Part model, mm, in its own coordinate system. Face numbers are marked on the shaded views. A direction names the side the tool comes from. Round coordinates to 2 decimals unless told otherwise and drop trailing zeros. Loops run counter-clockwise (first coordinate to the right, second up) from the corner with the lowest first, then second, coordinate; pieces in that order, holes last.
(1) Flat gauge pin, fed straight in: pin 1 (1 mm diameter, centred on x = -6, y = 6, fed in from +Z). Where does the tip first touch, or does it go through?
(2) Tool access for the marked faces 5 and 6: list every direction of +Z, -Z, +X, -X, +Y, -Y with a clear straight run to the whole face (end or side of a thin tool).
(3) Cut at D-D on z = -3. List the corners of the cut face in (x, y), then the cut area to 3 significant figures.
(4) Probe probe 1 along Z at (x, y) = (0, 43.6); probe 2 along X at (y, z) = (42.9, 0); probe 3 along Y at (x, z) = (7.75, -1.5). List the from-to ranges inside material, lowest first.
(5) Cut at A-A on x = 0. Count the separate pieces of the cut face and the enclosed holes in it, then the cut area to 3 significant figures.
(6) Mould opens along Y. For the marked faces 1, 2, 3 and 4 say: +Y half, -Y half, draft (parallel to the pull), parting line (faces both ways), or undercut.
(7) Cut at C-C on x = -9.5. List the corners of the cut face in (y, z), then the cut area to 3 significant figures.
from build123d import *

# Parameters (mm, degrees)
SKETCH1_R           = 4
BOSS_EXTRUDE1_DEPTH = 45.15
SKETCH2_W           = 40
SKETCH2_H           = 37.65
CUT_EXTRUDE1_DEPTH  = 26
SKETCH3_R           = 1.65
CUT_EXTRUDE2_DEPTH  = 46.15
CIRPATTERN1_COUNT   = 4
FILLET1_R           = 2


with BuildPart() as part:
    # Sketch1 → Boss-Extrude1 (new body)
    with BuildSketch(Plane(origin=(0, 0, 0), x_dir=(1, 0, 0), z_dir=(0, 1, 0))):
        with BuildLine():
            Line((-12.5, 15), (-12.5, 20))
            Line((-12.5, 20), (12.5, 20))
            Line((12.5, 20), (12.5, 15))
            Line((12.5, 15), (6.614378278, 7.5))
            ThreePointArc((6.614378278, 7.5), (0, -10), (-6.614378278, 7.5))
            Line((-6.614378278, 7.5), (-12.5, 15))
        make_face()
        Circle(SKETCH1_R, mode=Mode.SUBTRACT)
    extrude(amount=BOSS_EXTRUDE1_DEPTH)

    # Sketch2 → Cut-Extrude1 (cut, through all)
    with BuildSketch(Plane.ZY.offset(12.5)):
        with Locations((5, 22.575)):
            Rectangle(SKETCH2_W, SKETCH2_H)
    extrude(amount=-CUT_EXTRUDE1_DEPTH, mode=Mode.SUBTRACT)

    # Sketch3 → Cut-Extrude2 (cut, through all)
    with BuildSketch(Plane(origin=(0, 45.15, 0), x_dir=(1, 0, 0), z_dir=(0, 1, 0))):
        with Locations((0, 7)):
            Circle(SKETCH3_R)
    cut_extrude2 = extrude(amount=-CUT_EXTRUDE2_DEPTH, mode=Mode.SUBTRACT)

    # CirPattern1: Cut-Extrude2 ×4 about axis
    cirpattern1_axis = Axis((0, 0, 0), (0, 1, 0))
    for i in range(1, CIRPATTERN1_COUNT):
        add(cut_extrude2.rotate(cirpattern1_axis, i * 360 / CIRPATTERN1_COUNT), mode=Mode.SUBTRACT)

    # Fillet1
    fillet1_edges = [part.edges().sort_by_distance(p)[0] for p in [
        (6.614378278, 43.275, -7.5),
        (-6.614378278, 43.275, -7.5),
        (6.614378278, 1.875, -7.5),
        (-6.614378278, 1.875, -7.5),
    ]]
    fillet(fillet1_edges, radius=FILLET1_R)


solid = part.part
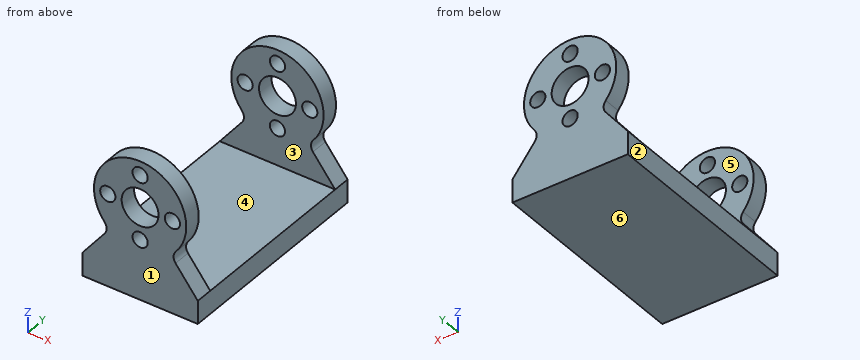
Final values:
1. pin 1: stops at z = -15
2. face 5: +Z, +X, -X
2. face 6: -Z, +X, -X, +Y, -Y
3. outline: (-9.54, 0) - (-2.65, 0) - (-2.65, 3.75) - (-9.54, 3.75) - close; (-9.54, 41.4) - (-2.65, 41.4) - (-2.65, 45.15) - (-9.54, 45.15) - close; (2.65, 0) - (9.54, 0) - (9.54, 3.75) - (2.65, 3.75) - close; (2.65, 41.4) - (9.54, 41.4) - (9.54, 45.15) - (2.65, 45.15) - close
3. area: 103 mm2
4. probe 1: z = -20 to -8.65, -5.35 to -4, 4 to 5.35, 8.65 to 10
4. probe 2: x = -10 to -8.65, -5.35 to -4, 4 to 5.35, 8.65 to 10
4. probe 3: y = 0 to 3.75, 41.4 to 45.15
5. separate pieces: 7
5. enclosed holes: 0
5. area: 304 mm2
6. face 1: -Y half
6. face 2: draft
6. face 3: undercut
6. face 4: undercut
7. outline: (0, -20) - (45.15, -20) - (45.15, -11.18) - (41.4, -11.18) - (41.4, -15) - (3.75, -15) - (3.75, -11.18) - (0, -11.18) - close; (0, -3.12) - (3.75, -3.12) - (3.75, 3.12) - (0, 3.12) - close; (41.4, -3.12) - (45.15, -3.12) - (45.15, 3.12) - (41.4, 3.12) - close
7. area: 301 mm2
